For this review, take the finished solid that the model builds, in its own axes (mm). Face numbers are marked on the shaded views. A direction names the side the tool comes from. Give positions to 0.01 mm unless a question says otherwise; leave off trailing zeros. Write each loop counter-clockwise with the first axis right and the second up, starting at its lowest first coordinate (ties: lowest second). Pieces come first, ordered by that corner, then holes. Notation, with made-up numbers: M 69,46 L 109,46 A18 cw 109,58 Z; hole C 21.25,18.25 d8. An arc over 180 degrees is marked long. Answer as a JSON object with one key per item and string values. Group by question number.
```python
from build123d import *

# Parameters (mm, degrees)
F0_R      = 7
F1_DEPTH  = 14.4
F4_DEPTH  = 10
F7_DEPTH  = 10
F8_DEPTH  = 6
F9_R      = 3.4
F10_DEPTH = 25
F11_R     = 4
F12_R     = 2


with BuildPart() as f1:
    # F0 (on Front) → F1 (new body, symmetric)
    with BuildSketch(Plane.XZ):
        with BuildLine():
            Line((100, 0), (12, 0))
            ThreePointArc((12, 0), (-8.4852813742, 8.4852813742), (0, -12))
            Line((0, -12), (100, -12))
            Line((100, -12), (100, 0))
        make_face()
        Circle(F0_R, mode=Mode.SUBTRACT)
    extrude(amount=F1_DEPTH, both=True)

    # F3 (on face) → F4 (join)
    with BuildSketch(Plane.XZ.offset(14.4)):
        with BuildLine():
            Line((65, 0), (75, 0))
            Line((75, 0), (75, 20))
            Line((75, 20), (65, 20))
            ThreePointArc((65, 20), (63.3288514808, 9.4820344172), (58.48, 0))
            Line((58.48, 0), (65, 0))
        make_face()
    extrude(amount=-F4_DEPTH)

    # F6 (on face) → F7 (cut)
    with BuildSketch(Plane.XZ.offset(14.4)):
        Polygon((58.3458282053, -12), (58.3458282053, 0), (43.7034219503, 0), (47.3529601204, -12), align=None)
    extrude(amount=-F7_DEPTH, mode=Mode.SUBTRACT)

    # F2 (on Front) → F8 (cut, symmetric)
    with BuildSketch(Plane.XZ):
        with BuildLine():
            Line((14, -12), (14, 0))
            Line((14, 0), (12, 0))
            ThreePointArc((12, 0), (-8.4852813742, 8.4852813742), (0, -12))
            Line((0, -12), (14, -12))
        make_face()
    extrude(amount=F8_DEPTH, both=True, mode=Mode.SUBTRACT)

    # F9 (on face) → F10 (cut)
    with BuildSketch(Plane.XY):
        with Locations((77, 5)):
            Circle(F9_R)
    extrude(amount=-F10_DEPTH, mode=Mode.SUBTRACT)

    # F11
    f11_edges = [f1.edges().sort_by_distance(p)[0] for p in [
        (100, 0, 0),
        (75, -9.4, 20),
    ]]
    fillet(f11_edges, radius=F11_R)

    # F12
    f12_edges = [f1.edges().sort_by_distance(p)[0] for p in [
        (75, -9.4, 0),
        (12, 10.2, 0),
        (12, -10.2, 0),
    ]]
    fillet(f12_edges, radius=F12_R)


solid = f1.part
```
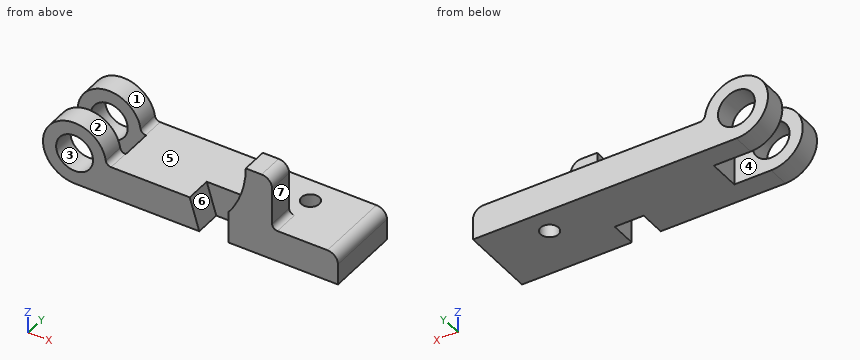
Item 1: Draft analysis for pull direction X (two halves, no side actions). For the marked faces 1, 2, 3 and 4, state which applies: released by +X, released by -X, zero draft, split by the parting line, or undercut.
Item 2: Consider section B-B (z = -6). Give the boundary of the cut face in (x, y), plus the area to 3 significant figures.
Item 3: Consider section A-A (y = 5). Give the boundary of the cut face in (x, z), plus the area to 3 significant figures.
Item 4: Machinability: for the marked faces 5, 6 and 7, which of the approach directions +Z, -Z, +X, -X, +Y, -Y give a long, thin tool a straight path to every point of the face, cutting with its end or side? Answer none if there is none.
Item 5: Consider section D-D (x = 10). Give the boundary of the cut face in (y, z), plus the area to 3 significant figures.
Item 6: Insertion check: P1, Ø1, axis at y = -4.5, z = 14.5, coming from the -X side; P2, Ø1.5, axis at x = 65, z = 11, coming from the +Y side; P3, Ø5, axis at y = -11.5, z = 7, coming from the +X side. Each pin has a flat end and moves straight along its axis. Give the tip position at first contact, or say it passes through.
Item 7: Consider section C-C (x = -2). Give the boundary of the cut face in (y, z).
Item 8: To check wall thickness, follow probe 1 along Y at (x, z) = (77, -5); probe 2 along Z at (x, y) = (0, -11); probe 3 along Z at (x, y) = (88, -11). State the ranges of each line that lie inside material, in increasing order.
Result set:
{
 "1": {"face 1": "split by the parting line", "face 2": "undercut", "face 3": "undercut", "face 4": "zero draft"},
 "2": {"outline": "M -10.39,-14.4 L -3.61,-14.4 L -3.61,-6 L -10.39,-6 Z; M -10.39,6 L -3.61,6 L -3.61,14.4 L -10.39,14.4 Z; M 3.61,-14.4 L 45.53,-14.4 L 45.53,-4.4 L 58.35,-4.4 L 58.35,-14.4 L 100,-14.4 L 100,14.4 L 3.61,14.4 L 3.61,6 L 14,6 L 14,-6 L 3.61,-6 Z; hole C 77,5 d6.8", "area": "2,600 mm^2"},
 "3": {"outline": "M 14,-12 L 73.6,-12 L 73.6,0 L 14,0 Z; M 80.4,-12 L 100,-12 L 100,-4 A4 ccw 96,0 L 80.4,0 Z", "area": "947 mm^2"},
 "4": {"face 5": "+Z, +Y", "face 6": "+Z, -Y", "face 7": "+Z, +X, +Y, -Y"},
 "5": {"outline": "M -14.4,-12 L -6,-12 L -6,6.63 L -14.4,6.63 Z; M 6,-12 L 14.4,-12 L 14.4,6.63 L 6,6.63 Z", "area": "313 mm^2"},
 "6": {"P1": "stops at x = 64.47", "P2": "stops at y = -4.4", "P3": "stops at x = 75"},
 "7": {"outline": "M -14.4,-11.83 L -6,-11.83 L -6,-6.71 L -14.4,-6.71 Z; M -14.4,6.71 L -6,6.71 L -6,11.83 L -14.4,11.83 Z; M 6,-11.83 L 14.4,-11.83 L 14.4,-6.71 L 6,-6.71 Z; M 6,6.71 L 14.4,6.71 L 14.4,11.83 L 6,11.83 Z"},
 "8": {"probe 1": "y = -14.4 to 1.6, 8.4 to 14.4", "probe 2": "z = -12 to -7, 7 to 12", "probe 3": "z = -12 to 0"}
}
